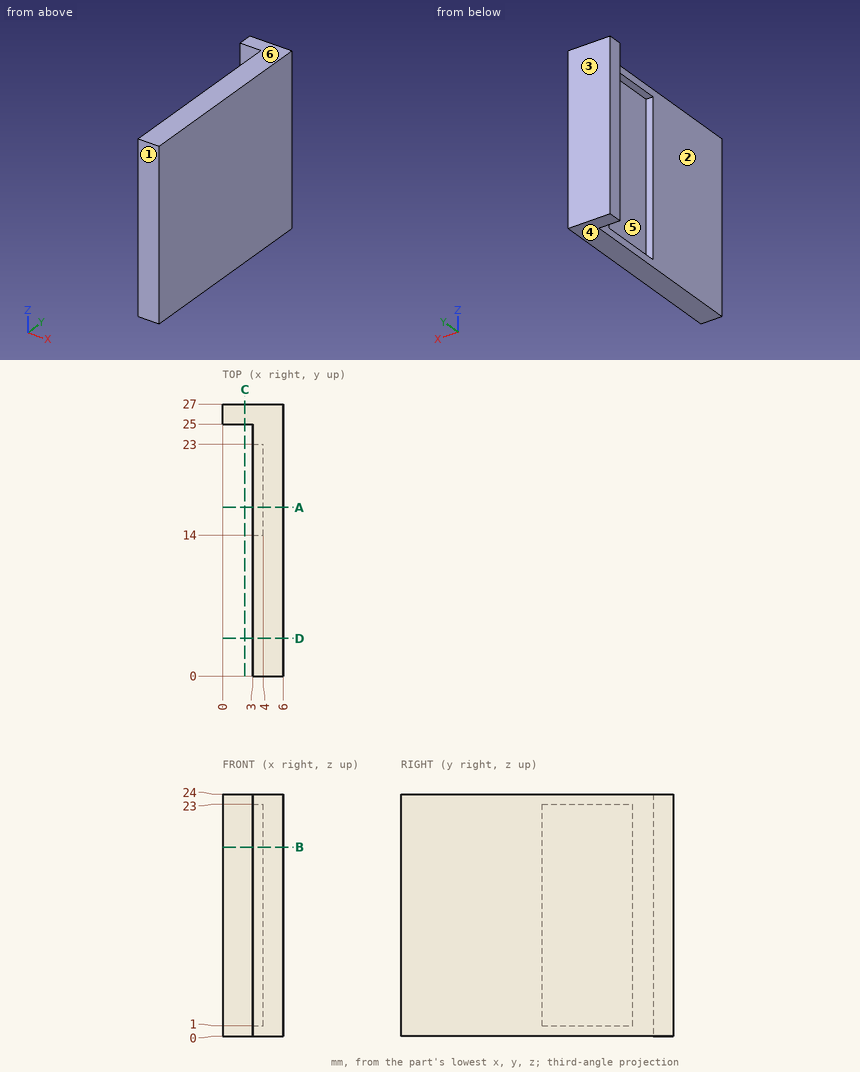
Can you work these out from the drawing? Everything is in mm from the part's minimum corner. A direction names the side the tool comes from. Give positions to 0.01 mm unless a question says otherwise; leave off trailing zeros. Write each loop counter-clockwise with the first axis right and the second up, starting at its lowest first coordinate (ties: lowest second). Pieces come first, ordered by that corner, then holes. Notation, with made-up numbers: M 14,36 L 39,36 A17 ccw 39,42 Z; hole C 19,2.5 d6. An arc over 180 degrees is marked long. Answer in a Markdown table with one row per item. Add a question column.
Item 1: On a 3-axis mill with a long thin cutter (end or side, diameter ignored), from which of +Z, -Z, +X, -X, +Y, -Y can I reach the whole of each face in a straight line? I mean the marked faces 1 and 2. Say none if no direction works.
Item 2: We'd pull the mould along Z, two halves only. Please class the marked faces 3, 4, 5 and 6: released by +Z, released by -Z, zero draft, split by the parting line, or undercut.
Item 3: Imagine slicing it at B-B, the plane z = 18.75. Write out the boundary of the cut face in (x, y).
Item 4: Imagine slicing it at D-D, the plane y = 3.75. Write out the boundary of the cut face in (x, z).
Item 5: Imagine slicing it at A-A, the plane y = 16.75. Write out the boundary of the cut face in (x, z), plus the area to 3 significant figures.
Item 6: Please list where these lines run through material, in increasing order: L1, parallel to Y at x = 3.2, z = 16; L2, parallel to Z at x = 3.55, y = 17.75; L3, parallel to X at y = 13.5, z = 2.5.
Item 7: Imagine slicing it at C-C, the plane x = 2.2. Write out the boundary of the cut face in (y, z), plus the area to 3 significant figures.
Item 8: For pin 1 Ø7 at (y, z) = (20, 11.5) entering from -X; pin 2 Ø1.5 at (x, z) = (1, 14) entering from -Y, each with a flat end and sliding along its axis, tell me the tip position at first contact or that it passes through.
Evaluation:
| question | item | result |
|---|---|---|
| 1 | face 1 | +Z, -Z, +X, -X, -Y |
| 1 | face 2 | +Z, -Z, -X, -Y |
| 2 | face 3 | zero draft |
| 2 | face 4 | released by -Z |
| 2 | face 5 | undercut |
| 2 | face 6 | released by +Z |
| 3 | outline | M 0,25 L 3,25 L 3,23 L 4,23 L 4,14 L 3,14 L 3,0 L 6,0 L 6,27 L 0,27 Z |
| 4 | outline | M 3,0 L 6,0 L 6,24 L 3,24 Z |
| 5 | outline | M 3,0 L 6,0 L 6,24 L 3,24 L 3,23 L 4,23 L 4,1 L 3,1 Z |
| 5 | area | 50.0 mm² |
| 6 | L1 | y = 0 to 14, 23 to 27 |
| 6 | L2 | z = 0 to 1, 23 to 24 |
| 6 | L3 | x = 3 to 6 |
| 7 | outline | M 25,0 L 27,0 L 27,24 L 25,24 Z |
| 7 | area | 48.0 mm² |
| 8 | pin 1 | stops at x = 3 |
| 8 | pin 2 | stops at y = 25 |
